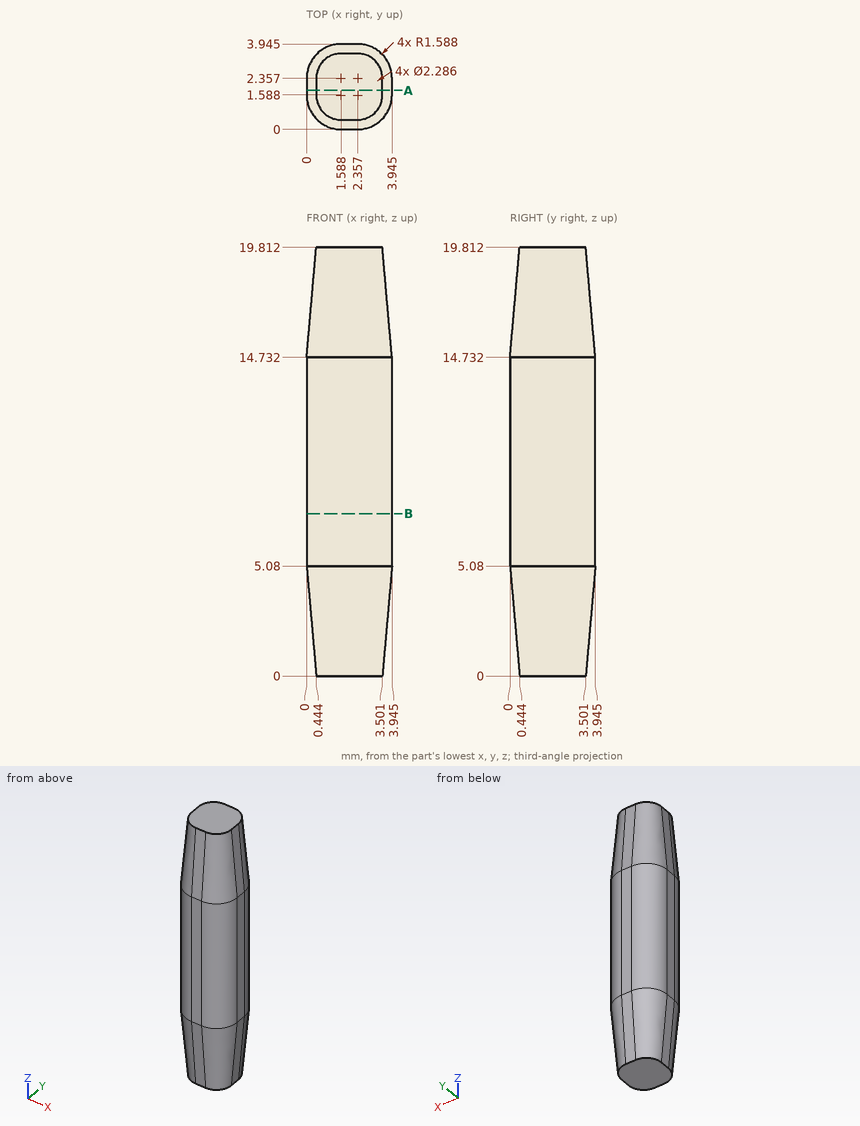
Here's the drawing with two shaded views (mm, measured from the low corner). I have some questions. Round coordinates to 2 decimals unless told otherwise and drop trailing zeros. Write each loop counter-clockwise with the first axis right and the second up, starting at its lowest first coordinate (ties: lowest second). Pieces come first, ordered by that corner, then holes. Notation, with made-up numbers: M -29,88.25 L 28,88.25 A32 cw 28,117.25 Z; hole C -16,-7.5 d11. An arc over 180 degrees is marked long. Answer in a Markdown table with one row per item. Add a question column.
Q1. Will this pin go through, and if not, where does the flat tip stop? pin 1 Ø1 at (x, z) = (3, 8.5) entering from -Y.
Q2. Imagine slicing it at A-A (y = 1.8). Please give me the cut outline in (x, z) (1 decimal).
Q3. Imagine slicing it at B-B (z = 7.5). Please give me the cut outline in (x, y) (1 decimal).
Q4. If I drill on line 1 (X direction, y = 1.5, z = 9.5); line 2 (X direction, y = 1, z = 13); line 3 (Y direction, x = 1.2, z = 12.5), over which ranges is the centre line in solid material (lowest first)? Write a range as from..to.
Values:
| question | item | result |
|---|---|---|
| 1 | pin 1 | y = 0.01 |
| 2 | outline | M 0,5.1 L 0.4,0 L 3.5,0 L 3.9,5.1 L 3.9,14.7 L 3.5,19.8 L 0.4,19.8 L 0,14.7 Z |
| 3 | outline | M 0,1.6 A1.6 ccw 1.6,0 L 2.4,0 A1.6 ccw 3.9,1.6 L 3.9,2.4 A1.6 ccw 2.4,3.9 L 1.6,3.9 A1.6 ccw 0,2.4 Z |
| 4 | line 1 | 0..3.94 |
| 4 | line 2 | 0.11..3.83 |
| 4 | line 3 | 0.05..3.9 |
